Verification items for the finished model (mm, model axes). Face numbers are marked on the shaded views. A direction names the side the tool comes from. Give positions to 0.01 mm unless a question says otherwise; leave off trailing zeros. Loops run counter-clockwise (first coordinate to the right, second up) from the corner with the lowest first, then second, coordinate; pieces in that order, holes last. Notation, with made-up numbers: (11, 81) - (51, 81) arc R24 cw to (51, 114) - close; hole circle Ø10 at (84.25, 84.5). An arc over 180 degrees is marked (long way). Answer in a Markdown table with one row per item.
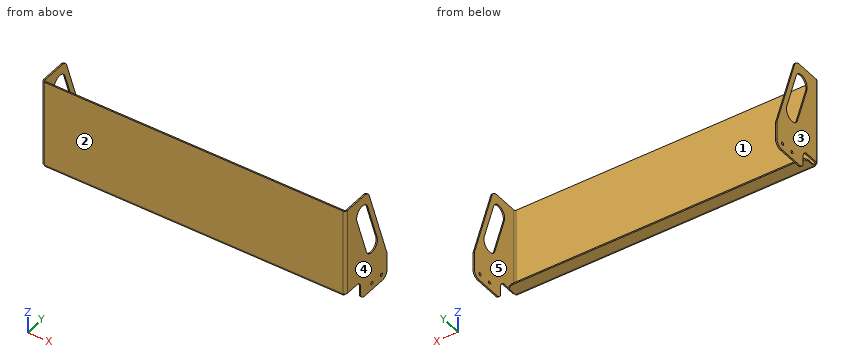
```python
from build123d import *

# Parameters (mm, degrees)
BASE_FLANGE1_DEPTH              = 203.2
SKETCH6_W                       = 44.40682
SKETCH6_H                       = 88.9
BOSS_EXTRUDE1_DEPTH             = 3.13182
SKETCH7_W                       = 44.40682
SKETCH7_H                       = 88.9
BOSS_EXTRUDE2_DEPTH             = 3.13182
CUT_EXTRUDE1_DEPTH              = 756.082359098
F_9_32_0_28125_DIAMETER_HOLE1_D = 7.14375
EDGE_FLANGE1_DEPTH              = 701.675
FILLET1_R                       = 12.7
FILLET2_R                       = 15.875


# Sheet-metal steps are written as plain solids
with BuildPart() as part:
    # Sketch1 → Base-Flange1 (new body)
    with BuildSketch(Plane.XY):
        with BuildLine():
            Line((-354.0125, 136.56818), (-354.0125, 3.175))
            ThreePointArc((-354.0125, 3.175), (-353.08256403, 0.92993597), (-350.8375, 0))
            Line((-350.8375, 0), (350.8375, 0))
            ThreePointArc((350.8375, 0), (353.08256403, 0.92993597), (354.0125, 3.175))
            Line((354.0125, 3.175), (354.0125, 136.56818))
            Line((354.0125, 136.56818), (357.14432, 136.56818))
            Line((357.14432, 136.56818), (357.14432, 3.175))
            ThreePointArc((357.14432, 3.175), (355.29709519, -1.28459519), (350.8375, -3.13182))
            Line((350.8375, -3.13182), (-350.8375, -3.13182))
            ThreePointArc((-350.8375, -3.13182), (-355.29709519, -1.28459519), (-357.14432, 3.175))
            Line((-357.14432, 3.175), (-357.14432, 136.56818))
            Line((-357.14432, 136.56818), (-354.0125, 136.56818))
        make_face()
    extrude(amount=BASE_FLANGE1_DEPTH)

    # Sketch6 → Boss-Extrude1 (add)
    with BuildSketch(Plane(origin=(357.14432, 0, 0), x_dir=(0, 0, -1), z_dir=(1, 0, 0))):
        with Locations((22.20341, 92.11818)):
            Rectangle(SKETCH6_W, SKETCH6_H)
    extrude(amount=-BOSS_EXTRUDE1_DEPTH)

    # Sketch7 → Boss-Extrude2 (add)
    with BuildSketch(Plane.ZY.offset(357.14432)):
        with Locations((-22.20341, 92.11818)):
            Rectangle(SKETCH7_W, SKETCH7_H)
    extrude(amount=-BOSS_EXTRUDE2_DEPTH)

    # Sketch8 → Cut-Extrude1 (cut, through all)
    with BuildSketch(Plane.ZY.offset(357.14432)):
        with BuildLine():
            Line((72.133349274, 103.379689668), (168.517386933, 71.244393115))
            ThreePointArc((168.517386933, 71.244393115), (180.56402589, 47.14701795), (156.466650726, 35.100378992))
            Line((156.466650726, 35.100378992), (60.082613067, 67.235675546))
            ThreePointArc((60.082613067, 67.235675546), (48.03597411, 91.333050711), (72.133349274, 103.379689668))
        make_face()
        Polygon((12.74318, 136.56818), (203.2, 73.06818), (203.2, 136.56818), align=None)
    extrude(amount=-CUT_EXTRUDE1_DEPTH, mode=Mode.SUBTRACT)

    # 9/32 (0.28125) Diameter Hole1 (through all)
    with Locations(Plane.ZY.offset(357.14432)):
        with Locations((-28.53182, 85.76818), (-28.53182, 117.51818)):
            Hole(F_9_32_0_28125_DIAMETER_HOLE1_D / 2)

    # Edge-Flange1 section (across the edge) → Edge-Flange1 (add)
    with BuildSketch(Plane(origin=(350.8375, 0, -3.175), x_dir=(0, 0, 1), z_dir=(-1, 0, 0))):
        with BuildLine():
            Line((-3.13182, 3.175), (-3.13182, 31.75))
            Line((-3.13182, 31.75), (0, 31.75))
            Line((0, 31.75), (0, 3.175))
            ThreePointArc((0, 3.175), (0.92993597, 0.92993597), (3.175, 0))
            Line((3.175, 0), (3.175, -3.13182))
            ThreePointArc((3.175, -3.13182), (-1.28459519, -1.28459519), (-3.13182, 3.175))
        make_face()
    extrude(amount=EDGE_FLANGE1_DEPTH)

    # Fillet1
    fillet1_edges = [part.edges().sort_by_distance(p)[0] for p in [
        (350.8375, 31.75, -4.74091),
        (-350.8375, 31.75, -4.74091),
        (355.57841, 47.66818, -44.40682),
        (355.57841, 47.66818, 0),
        (-355.57841, 47.66818, 0),
        (-355.57841, 47.66818, -44.40682),
    ]]
    fillet(fillet1_edges, radius=FILLET1_R)

    # Fillet2
    fillet2_edges = [part.edges().sort_by_distance(p)[0] for p in [
        (355.57841, 136.56818, -44.40682),
        (-355.57841, 136.56818, -44.40682),
        (-355.57841, 73.06818, 203.2),
        (355.57841, 73.06818, 203.2),
        (355.57841, 136.56818, 12.74318),
        (-355.57841, 136.56818, 12.74318),
    ]]
    fillet(fillet2_edges, radius=FILLET2_R)


solid = part.part
```
Q1. Draft check along X on the marked faces 1, 2 and 3. Enter one of: +X half, -X half, draft (parallel to the pull), parting line (faces both ways), or undercut.
Completed:
| item | result |
|---|---|
| face 1 | undercut |
| face 2 | draft |
| face 3 | -X half |
Q2. Sectioned sample at B-B (x = -174). Record the cut outline in (y, z) (3 decimals).
Completed:
| item | result |
|---|---|
| outline | (-3.132, 0) arc R6.307 ccw to (3.175, -6.307) - (31.75, -6.307) - (31.75, -3.175) - (3.175, -3.175) arc R3.175 cw to (0, 0) - (0, 203.2) - (-3.132, 203.2) - close |
Q3. Sectioned sample at A-A (z = 104). Give the number of separate pieces and of enclosed holes in the cut face, and give its area (3 significant figures).
Completed:
| item | result |
|---|---|
| separate pieces | 3 |
| enclosed holes | 0 |
| area | 2,640 mm^2 |
Q4. Go/stop test with flat-tipped pins: P1, Ø1.9, axis at x = 355, y = 17, coming from the -Z side; P2, Ø9.5, axis at y = 85.77, z = -28.53, coming from the -X side; P3, Ø3, axis at y = 9, z = -4.5, coming from the +X side; P4, Ø23, axis at x = 27.5, y = 17, coming from the +Z side (3 decimals). Record where each tip stops, or that it passes through.
Completed:
| item | result |
|---|---|
| P1 | z = 0 |
| P2 | x = -357.14 |
| P3 | x = 350.84 |
| P4 | z = -3.175 |
Q5. Tool access check on the marked faces 4 and 5. Record the directions out of +Z, -Z, +X, -X, +Y, -Y that give a thin tool (end or side, any length) a straight path to the whole face; none if there is none.
Completed:
| item | result |
|---|---|
| face 4 | +Z, -Z, +X, +Y, -Y |
| face 5 | +Z, -Z, +Y |
Q6. Thickness scan on line 1 (X direction, y = 96, z = -17); line 2 (Y direction, x = -61.5, z = 133); line 3 (Z direction, x = 122.5, y = 24) (3 decimals). Record the ranges inside material, lowest first.
Completed:
| item | result |
|---|---|
| line 1 | -357.14 to -354.01, 354.01 to 357.14 |
| line 2 | -3.13 to 0 |
| line 3 | -6.307 to -3.175 |
